Geometry: final body of the model. Coordinates: model frame, mm. Give positions to 0.01 mm unless a question says otherwise; leave off trailing zeros. Write each loop counter-clockwise with the first axis right and the second up, starting at its lowest first coordinate (ties: lowest second). Pieces come first, ordered by that corner, then holes.
from build123d import *

# Parameters (mm, degrees)
Y_KSEKLIK_EKSTR_ZYON1_DEPTH = 10
IZIM2_R                     = 2.5
KES_EKSTR_ZYON1_DEPTH       = 170


with BuildPart() as part:
    # Çizim1 → Yükseklik-Ekstrüzyon1 (new body)
    with BuildSketch(Plane(origin=(0, 0, 0), x_dir=(1, 0, 0), z_dir=(0, 1, 0))):
        with BuildLine():
            Line((-48.769745033, 34.22514167), (94.301322779, 34.22514167))
            ThreePointArc((94.301322779, 34.22514167), (95.715536341, 33.639355233), (96.301322779, 32.22514167))
            Line((96.301322779, 32.22514167), (96.301322779, 19.154073858))
            ThreePointArc((96.301322779, 19.154073858), (95.715536341, 17.739860296), (94.301322779, 17.154073858))
            Line((94.301322779, 17.154073858), (-48.769745033, 17.154073858))
            ThreePointArc((-48.769745033, 17.154073858), (-50.183958595, 17.739860296), (-50.769745033, 19.154073858))
            Line((-50.769745033, 19.154073858), (-50.769745033, 32.22514167))
            ThreePointArc((-50.769745033, 32.22514167), (-50.183958595, 33.639355233), (-48.769745033, 34.22514167))
        make_face()
    extrude(amount=Y_KSEKLIK_EKSTR_ZYON1_DEPTH)

    # Çizim2 → Kes-Ekstrüzyon1 (cut)
    with BuildSketch(Plane(origin=(96.301322779, 0, 0), x_dir=(0, 0, -1), z_dir=(1, 0, 0))):
        with Locations((25.689607764, 5)):
            Circle(IZIM2_R)
    extrude(amount=-KES_EKSTR_ZYON1_DEPTH, mode=Mode.SUBTRACT)


solid = part.part
Q1. Section B-B on x = -8. Output: boundary loops of the cut face in (y, z), plus the area to 3 significant figures.
Filled sheet:
outline: (0, -34.23) - (10, -34.23) - (10, -17.15) - (0, -17.15) - close; hole circle Ø5 at (5, -25.69)
area: 151 mm2
Q2. Ray query, line 1 along Y through (x, z) = (60.5, -26); line 2 along Z through (x, y) = (38, 6.5); line 3 along X through (y, z) = (7.25, -19). Return the intervals inside material, ascending.
Filled sheet:
line 1: y = 0 to 2.52, 7.48 to 10
line 2: z = -34.23 to -27.69, -23.69 to -17.15
line 3: x = -50.76 to 96.3
Q3. Pin query (flat end, axial travel): P1, Ø6, axis at y = 1, z = -19, coming from the -X side. Return the tip coordinate at first contact, or that it passes through.
Filled sheet:
P1: stops at x = -50.77
Q4. Section C-C on z = -27. Output: boundary loops of the cut face in (x, y), plus the area to 3 significant figures.
Filled sheet:
outline: (-50.77, 0) - (96.3, 0) - (96.3, 2.87) - (-50.77, 2.87) - close; (-50.77, 7.13) - (96.3, 7.13) - (96.3, 10) - (-50.77, 10) - close
area: 844 mm2
Q5. Section A-A on y = 5. Output: boundary loops of the cut face in (x, z).
Filled sheet:
outline: (-50.77, -32.23) arc R2 ccw to (-48.77, -34.23) - (94.3, -34.23) arc R2 ccw to (96.3, -32.23) - (96.3, -28.19) - (-50.77, -28.19) - close; (-50.77, -23.19) - (96.3, -23.19) - (96.3, -19.15) arc R2 ccw to (94.3, -17.15) - (-48.77, -17.15) arc R2 ccw to (-50.77, -19.15) - close
Q6. Pull-direction query (Z, two-part tool) for faces 1 (the cylindrical face through (23.8, 6.69, -23.85)), 2 (the flat face through (-50.77, 2.7, -24.1)), 3 (the flat face through (24, 5, -17.154)); classes: released by +Z, released by -Z, zero draft, split by the parting line, or undercut.
Filled sheet:
face 1: undercut
face 2: zero draft
face 3: released by +Z
